For this review, take the finished solid that the model builds, in its own axes (mm). A direction names the side the tool comes from. Coordinates: 2 decimals unless noted, no trailing zeros. Loops run counter-clockwise (first coordinate to the right, second up) from the corner with the lowest first, then second, coordinate; pieces in that order, holes last. Notation, with made-up numbers: (6.5, -4) -> (40.5, -4) arc R13 cw to (40.5, 2) -> close; hole circle Ø8 at (30.25, 46.25). An arc over 180 degrees is marked (long way). Use a Markdown table: item, result.
Autodesk Inventor part; units mm, degrees
ref_plane "YZ Plane" through (0, 0, 0) normal (1, 0, 0) x (0, 1, 0)
ref_plane "XZ Plane" through (0, 0, 0) normal (0, 1, 0) x (-1, 0, 0)
ref_plane "XY Plane" through (0, 0, 0) normal (0, 0, 1) x (1, 0, 0)
sketch "Sketch1" plane through (0, 0, 0) normal (0, 0, 1) x (1, 0, 0)
  circle A0 centre (0, 0) radius 4
  dimension "d0" = 8
extrude "Extrusion1" add sketch "Sketch1" against normal blind 11.7
sketch "Sketch2" plane through (0, 0, 0) normal (0, 0, 1) x (1, 0, 0)
  circle A0 centre (0, 0) radius 4
  circle A1 centre (0, 0) radius 3
  dimension "d3" = 6
extrude "Extrusion2" add sketch "Sketch2" along normal blind 4.5 contours A1
thread "Thread1"
sketch "Sketch3" plane through (0, 0, 4.5) normal (0, 0, 1) x (1, 0, 0)
  circle A0 centre (0, 0) radius 3
  circle A1 centre (0, 0) radius 1.8
  dimension "d8" = 3.6
extrude "Extrusion3" cut sketch "Sketch3" against normal blind 15 contours A1
sketch "Sketch4" plane through (0, 0, -11.7) normal (0, 0, -1) x (-1, 0, 0)
  circle A0 centre (0, 0) radius 4 construction
  line L0 (0, 0) -> (0, 2.7273) construction
  line L1 (-2.5, 1) -> (-2, 1)
  line L2 (-2, 1) -> (-2, -1)
  line L3 (-2, -1) -> (-2.5, -1)
  line L4 (-2.5, -1) -> (-2.5, 1)
  line L5 (2.5, 1) -> (2, 1)
  line L6 (2, 1) -> (2, -1)
  line L7 (2, -1) -> (2.5, -1)
  line L8 (2.5, -1) -> (2.5, 1)
  dimension "d11" = 2
  dimension "d12" = 0.5
  dimension "d13" = 2
  dimension "d14" = 1
extrude "Extrusion4" add sketch "Sketch4" along normal blind 3
sketch "Sketch5" plane through (0, 0, -11.7) normal (0, 0, -1) x (-1, 0, 0)
  circle A0 centre (0, 0) radius 4
  line L0 (-1, 2) -> (1, 2)
  line L1 (1, 2) -> (1, 2.5)
  line L2 (1, 2.5) -> (-1, 2.5)
  line L3 (-1, 2.5) -> (-1, 2)
  line L4 (-1, 2) -> (1, 2.5) construction
  line L5 (1, 2) -> (-1, 2.5) construction
  point P0 (0, 2.25)
  dimension "d17" = 2
  dimension "d18" = 0.5
  dimension "d19" = 2
  dimension "d20" = 1
extrude "Extrusion5" add sketch "Sketch5" along normal blind 6.1 contours L3 L2 L1 L0
sketch "Sketch6" plane through (2.5, -1, -11.7) normal (1, 0, 0) x (0, 0, -1)
  line L0 (3, 2) -> (3, 0)
  circle A0 centre (2, 1) radius 0.5
  point P0 (-11.7, 1)
  dimension "d23" = 1
  dimension "d24" = 1
extrude "Extrusion6" cut sketch "Sketch6" against normal through all
sketch "Sketch7" plane through (-1, 2.5, -11.7) normal (0, 1, 0) x (1, 0, 0)
  line L0 (0, 6.1) -> (2, 6.1)
  circle A0 centre (1, 5.1) radius 0.5
  point P0 (1, -11.7)
  dimension "d27" = 1
  dimension "d28" = 1
extrude "Extrusion7" cut sketch "Sketch7" against normal blind 6.1
sketch "Sketch8" plane through (2.5, -1, -11.7) normal (1, 0, 0) x (0, 0, -1)
  circle A0 centre (2, 1) radius 0.5
sketch "Sketch9" plane through (-1, 2, -11.7) normal (0, -1, 0) x (1, 0, 0)
  circle A0 centre (1, -5.1) radius 0.5
sketch "Sketch10" plane through (-2.5, -1, -11.7) normal (-1, 0, 0) x (0, 0, 1)
  circle A0 centre (-2, 1) radius 0.5
equation "\"d14\" = 0.5 * d11"
equation "\"d20\" = 0.5 * d17"
properties part number "MJ-074N" material "Nickel-Copper Alloy 400"
(1) Mouldability with a two-part tool opening along Z and no side actions: class faces 1 (the face through (2.254, 0.15, -14.177)), 2 (the face through (0, 0, -10.5)), 3 (the face through (-2.5, 0, -13)) as pulls with the +Z half, pulls with the -Z half, needs draft (parallel to the pull), parting line crosses it, or undercut.
Found:
| item | result |
|---|---|
| face 1 | undercut |
| face 2 | pulls with the +Z half |
| face 3 | needs draft |
(2) Take a section at D-D on z = -1.5. Write out the cut boundary in (x, y).
Found:
| item | result |
|---|---|
| outline | circle Ø8 at (0, 0); hole circle Ø3.6 at (0, 0) |
(3) Take a section at A-A on z = -16.8. Write out the cut boundary in (x, y).
Found:
| item | result |
|---|---|
| outline | (-1, 2) -> (-0.5, 2) -> (-0.5, 2.5) -> (-1, 2.5) -> close; (0.5, 2) -> (1, 2) -> (1, 2.5) -> (0.5, 2.5) -> close |
(4) For line 1 along Y through (x, z) = (0, -6.5); line 2 along Y through (x, z) = (-2.4, -13.7); line 3 along Z through (x, y) = (-0.5, 0.25), list the stretches that pass through material, from the lowest coordinate up.
Found:
| item | result |
|---|---|
| line 1 | y = -4 to -1.8, 1.8 to 4 |
| line 2 | y = -1 to -0.5, 0.5 to 1 |
| line 3 | z = -11.7 to -10.5 |
(5) For pin 1 Ø1.1 at (x, y) = (0.5, -0.5) entering from +Z; pin 2 Ø1.5 at (y, z) = (-3, -4) entering from +X; pin 3 Ø0.6 at (x, y) = (-2, -0.5) entering from -Z, all flat-tipped, find the tip position at first contact; note any pin that passes through.
Found:
| item | result |
|---|---|
| pin 1 | stops at z = -10.5 |
| pin 2 | stops at x = 3.31 |
| pin 3 | stops at z = -14.7 |
(6) For faces 4 (the face through (1, 3, 0)), 5 (the face through (0, 2.5, -15)), 6 (the face through (0, 2, -15)), list the 3-axis set-ups (+Z, -Z, +X, -X, +Y, -Y) from which the entire face can be reached by the end or side of a thin tool; tool diameter is ignored.
Found:
| item | result |
|---|---|
| face 4 | +Z |
| face 5 | -Z, +X, -X, +Y |
| face 6 | -Z, +X, -X, -Y |
(7) Take a section at C-C on x = 0. Write out the cut boundary in (y, z), plus the area to 4 significant figures.
Found:
| item | result |
|---|---|
| outline | (-4, -11.7) -> (2, -11.7) -> (2, -16.3) -> (2.5, -16.3) -> (2.5, -11.7) -> (4, -11.7) -> (4, 0) -> (3, 0) -> (3, 4.5) -> (1.8, 4.5) -> (1.8, -10.5) -> (-1.8, -10.5) -> (-1.8, 4.5) -> (-3, 4.5) -> (-3, 0) -> (-4, 0) -> close; (2, -17.8) -> (2.5, -17.8) -> (2.5, -17.3) -> (2, -17.3) -> close |
| area | 69.15 mm^2 |
(8) Take a section at B-B on y = 0. Write out the cut boundary in (x, z), plus the area to 3 significant figures.
Found:
| item | result |
|---|---|
| outline | (-4, -11.7) -> (-2.5, -11.7) -> (-2.5, -13.2) -> (-2, -13.2) -> (-2, -11.7) -> (2, -11.7) -> (2, -13.2) -> (2.5, -13.2) -> (2.5, -11.7) -> (4, -11.7) -> (4, 0) -> (3, 0) -> (3, 4.5) -> (1.8, 4.5) -> (1.8, -10.5) -> (-1.8, -10.5) -> (-1.8, 4.5) -> (-3, 4.5) -> (-3, 0) -> (-4, 0) -> close; (-2.5, -14.7) -> (-2, -14.7) -> (-2, -14.2) -> (-2.5, -14.2) -> close; (2, -14.7) -> (2.5, -14.7) -> (2.5, -14.2) -> (2, -14.2) -> close |
| area | 68.6 mm^2 |
